from build123d import *

# Parameters (mm, degrees)
F0_W     = 70
F0_H     = 10
F1_DEPTH = 8
F2_W     = 58
F2_H     = 10
F3_DEPTH = 12
F5_DEPTH = 7.5
F7_D     = 4.4
F8_DEPTH = 2
F9_R     = 1
F10_R    = 2


with BuildPart() as f1:
    # F0 (on Top) → F1 (new body)
    with BuildSketch(Plane.XY):
        Rectangle(F0_W, F0_H)
    extrude(amount=F1_DEPTH)

    # F2 (on face) → F3 (join)
    with BuildSketch(Plane.XY.offset(8)):
        with Locations((6, 0)):
            Rectangle(F2_W, F2_H)
    extrude(amount=F3_DEPTH)

    # F4 (on Front) → F5 (cut, symmetric)
    with BuildSketch(Plane.XZ):
        with BuildLine():
            ThreePointArc((0, 5), (12.3743686708, 10.1256313292), (17.5, 22.5))
            ThreePointArc((17.5, 22.5), (17.4550693399, 23.7532175939), (17.3205080757, 25))
            ThreePointArc((17.3205080757, 25), (-13.2287565553, 33.9564392374), (0, 5))
        make_face()
        with BuildLine():
            ThreePointArc((17.3205080757, 25), (17.4550693399, 23.7532175939), (17.5, 22.5))
            ThreePointArc((17.5, 22.5), (12.3743686708, 10.1256313292), (0, 5))
            Line((0, 5), (17.1464281995, 5))
            ThreePointArc((17.1464281995, 5), (22.5869153592, 13.0088854945), (24.5, 22.5))
            ThreePointArc((24.5, 22.5), (24.4680079159, 23.7516343834), (24.3721152139, 25))
            Line((24.3721152139, 25), (17.3205080757, 25))
        make_face()
        with BuildLine():
            Line((36.3039560616, 25), (24.3721152139, 25))
            ThreePointArc((24.3721152139, 25), (24.4680079159, 23.7516343834), (24.5, 22.5))
            ThreePointArc((24.5, 22.5), (22.5869153592, 13.0088854945), (17.1464281995, 5))
            Line((17.1464281995, 5), (36.3039560616, 5))
            Line((36.3039560616, 5), (36.3039560616, 25))
        make_face()
    extrude(amount=F5_DEPTH, both=True, mode=Mode.SUBTRACT)

    # F7 (through all)
    with Locations(Plane.XY.offset(8)):
        with Locations((-29, 0), (29, 0)):
            Hole(F7_D / 2)

    # F4 (on Front) → F8 (cut, symmetric)
    with BuildSketch(Plane.XZ):
        with BuildLine():
            ThreePointArc((0, 5), (-13.2287565553, 33.9564392374), (17.3205080757, 25))
            Line((17.3205080757, 25), (24.3721152139, 25))
            ThreePointArc((24.3721152139, 25), (-14.008418473, 42.600104773), (-10.7819293264, 0.5))
            Line((-10.7819293264, 0.5), (10.7819293264, 0.5))
            ThreePointArc((10.7819293264, 0.5), (14.1442846593, 2.4952702724), (17.1464281995, 5))
            Line((17.1464281995, 5), (0, 5))
        make_face()
        with BuildLine():
            ThreePointArc((17.3205080757, 25), (17.4550693399, 23.7532175939), (17.5, 22.5))
            ThreePointArc((17.5, 22.5), (12.3743686708, 10.1256313292), (0, 5))
            Line((0, 5), (17.1464281995, 5))
            ThreePointArc((17.1464281995, 5), (22.5869153592, 13.0088854945), (24.5, 22.5))
            ThreePointArc((24.5, 22.5), (24.4680079159, 23.7516343834), (24.3721152139, 25))
            Line((24.3721152139, 25), (17.3205080757, 25))
        make_face()
    extrude(amount=F8_DEPTH, both=True, mode=Mode.SUBTRACT)

    # F9
    f9_edges = [f1.edges().sort_by_distance(p)[0] for p in [
        (-17.320508, 3.5, 20),
        (-17.320508, -3.5, 20),
        (-23, -3.5, 20),
        (-23, 3.5, 20),
        (-23, 0, 14.059028),
    ]]
    fillet(f9_edges, radius=F9_R)

    # F10
    f10_edges = [f1.edges().sort_by_distance(p)[0] for p in [
        (-35, -5, 4),
        (-35, 5, 4),
        (35, -5, 2.5),
        (35, 5, 2.5),
    ]]
    fillet(f10_edges, radius=F10_R)


solid = f1.part
For this review, take the finished solid that the model builds, in its own axes (mm). A direction names the side the tool comes from. Coordinates: 2 decimals unless noted, no trailing zeros. Order: outer loops, then holes, each group sorted by start corner. A loop starts at its lowest first (then second) coordinate and runs counter-clockwise, first axis right, second up. Notation, with made-up numbers: (-23, 82.25) - (-14, 82.25) arc R14 ccw to (-14, 104.25) - close; hole circle Ø11 at (37.5, 15.25). An arc over 180 degrees is marked (long way). Answer as CSV lines item,"result". Start each with the question number.
1) Add section B-B (y = 0). State the section outline as (x, z) points.
2) Draft analysis for pull direction X (two halves, no side actions). For faces 1 (the cylindrical face through (31.198, 0.097, 2.465)), 2 (the cylindrical face through (-34.43, 4.4, 4.06)), 3 (the cylindrical face through (-11.27, 3.48, 9.11)), state which applies: +X half, -X half, draft (parallel to the pull), parting line (faces both ways), or undercut.
3) Add section A-A (x = 29). State the section outline as (y, z) points.
4) Add section C-C (z = 16). State the section outline as (x, y) points.
5) Machinability: for faces 4 (the flat face through (0, 0, 0.5)), 5 (the flat face through (-27.8, -2.2, 8)), 6 (the flat face through (-20, -3, 20)), which of the approach directions +Z, -Z, +X, -X, +Y, -Y give a long, thin tool a straight path to every point of the face, cutting with its end or side? Answer none if there is none.
6) To check wall thickness, follow line 1 along Y through (x, z) = (29, 1.65); line 2 along Y through (x, z) = (-19, 9); line 3 along Z through (x, y) = (-22, -0.5). State the ranges of each line that lie inside material, in increasing order. Write a range as [from, to].
7) Insertion check: P1, Ø4, axis at y = -1, z = 17.5, coming from the -X side; P2, Ø6, axis at y = -2.5, z = 15.5, coming from the +X side; P3, Ø3, axis at x = -27.5, y = 0.5, coming from the +Z side; P4, Ø4, axis at x = -29, y = 0, coming from the -Z side. Each pin has a flat end and moves straight along its axis. Give the tip position at first contact, or say it passes through.
8) Add section D-D (x = 9). State the section outline as (y, z) points.
Result:
1,outline,"(-35, 0) - (-31.2, 0) - (-31.2, 8) - (-35, 8) - close; (-26.8, 0) - (26.8, 0) - (26.8, 5) - (17.15, 5) arc R24.5 cw to (10.78, 0.5) - (-10.78, 0.5) arc R24.5 cw to (-21.14, 10.11) arc R1 ccw to (-23, 9.61) - (-23, 8) - (-26.8, 8) - close; (31.2, 0) - (35, 0) - (35, 5) - (31.2, 5) - close"
2,face 1,"undercut"
2,face 2,"-X half"
2,face 3,"+X half"
3,outline,"(-5, 0) - (-2.2, 0) - (-2.2, 5) - (-5, 5) - close; (2.2, 0) - (5, 0) - (5, 5) - (2.2, 5) - close"
4,outline,"(-23, -5) - (-16.25, -5) - (-16.25, -2) - (-23, -2) - close; (-23, 2) - (-16.25, 2) - (-16.25, 5) - (-23, 5) - close"
5,face 4,"+Z"
5,face 5,"+Z, -X, +Y, -Y"
5,face 6,"+Z, +X, -X, +Y, -Y"
6,line 1,"[-5, -2.2], [2.2, 5]"
6,line 2,"[-5, -2], [2, 5]"
6,line 3,"[0, 10.61]"
7,P1,"x = -23"
7,P2,"x = -14.36"
7,P3,"z = 8"
7,P4,"through"
8,outline,"(-5, 0) - (5, 0) - (5, 5) - (2, 5) - (2, 0.5) - (-2, 0.5) - (-2, 5) - (-5, 5) - close"
